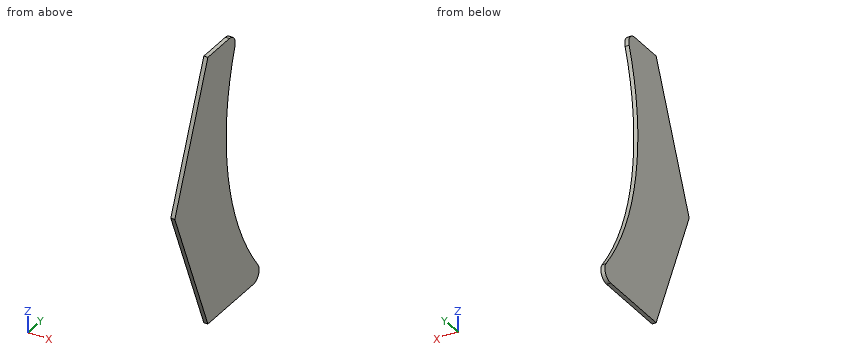
```python
from build123d import *

# Parameters (mm, degrees)
F1_DEPTH = 2.5


with BuildPart() as f1:
    # F0 (on Right) → F1 (new body)
    with BuildSketch(Plane.YZ):
        with BuildLine():
            ThreePointArc((-3.018316, 75.444877), (-3.793379, 80.894136), (-8.684346, 83.418731))
            Line((-8.684346, 83.418731), (-30.6, 83.418731))
            Line((-30.6, 83.418731), (-64.303355, 0))
            Line((-64.303355, 0), (-30.6, -83.418731))
            Line((-30.6, -83.418731), (15.726308, -83.418731))
            ThreePointArc((15.726308, -83.418731), (21.098828, -80.090065), (20.510239, -73.797405))
            ThreePointArc((20.510239, -73.797405), (-9.973866, -2.127509), (-3.018316, 75.444877))
        make_face()
    extrude(amount=F1_DEPTH)


solid = f1.part
```
Work out the finished part from the listing and answer in its coordinate system (mm). Round coordinates to 2 decimals unless told otherwise and drop trailing zeros. Order: outer loops, then holes, each group sorted by start corner. A loop starts at its lowest first (then second) coordinate and runs counter-clockwise, first axis right, second up.
Q1. A cutting plane is placed at A-A, the plane x = 2. Determine the outline of the cut face in (y, z), then the cut area to 3 significant figures.
Solution:
outline: (-64.3, 0) - (-30.6, -83.42) - (15.73, -83.42) arc R6 ccw to (20.51, -73.8) arc R160.04 cw to (-3.02, 75.44) arc R6 ccw to (-8.68, 83.42) - (-30.6, 83.42) - close
area: 7,460 mm2
Q2. A cutting plane is placed at C-C, the plane y = -33. Determine the outline of the cut face in (x, z), then the cut area to 3 significant figures.
Solution:
outline: (0, -77.48) - (2.5, -77.48) - (2.5, 77.48) - (0, 77.48) - close
area: 387 mm2
Q3. Find the intervals of material crossed by line 1 along Y through (x, z) = (0.75, 28.5); line 2 along Z through (x, y) = (0.35, -61); line 3 along Y through (x, z) = (2, 56), in increasing order.
Solution:
line 1: y = -52.79 to -11.82
line 2: z = -8.18 to 8.18
line 3: y = -41.68 to -8.44
Q4. A cutting plane is placed at B-B, the plane z = 3. Determine the outline of the cut face in (x, y), then the cut area to 3 significant figures.
Solution:
outline: (0, -63.09) - (2.5, -63.09) - (2.5, -10.7) - (0, -10.7) - close
area: 131 mm2
